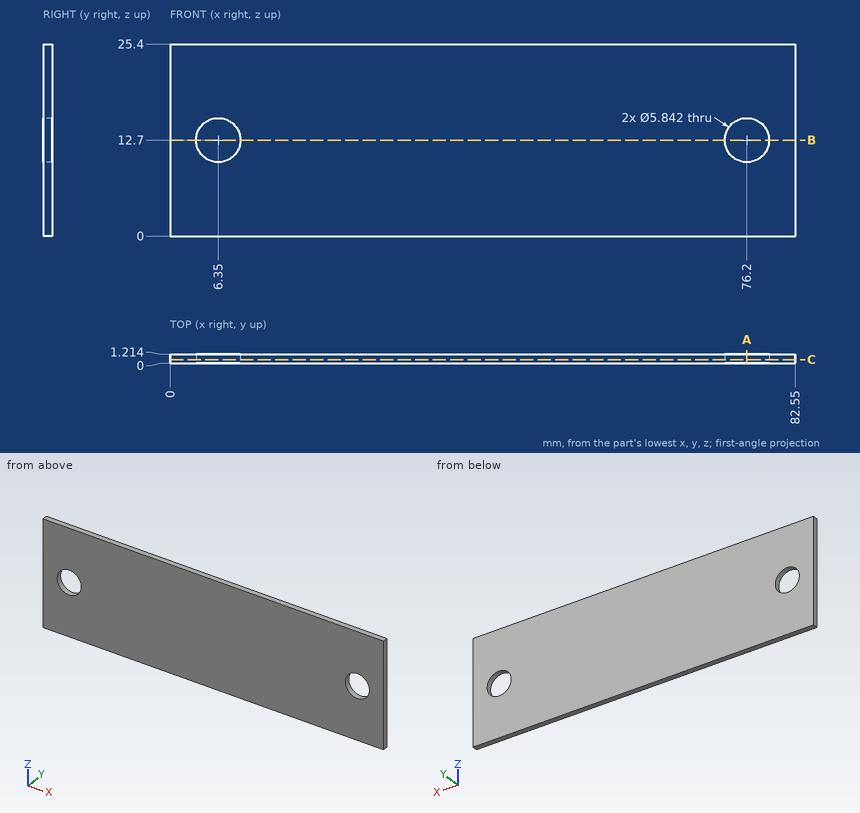
The drawing under review shows one solid part. Ordinate dimensions are in mm from its lowest x, y, z. Round coordinates to 2 decimals unless told otherwise and drop trailing zeros. Order: outer loops, then holes, each group sorted by start corner. A loop starts at its lowest first (then second) coordinate and runs counter-clockwise, first axis right, second up. Notation, with made-up numbers: M 61.25,7 L 110.25,7 A21 ccw 110.25,40 Z; hole C -35.75,-38.75 d6. An arc over 180 degrees is marked long. Answer as CSV lines item,"result". Start each with the question number.
1) Add section C-C (y = 0.5). Give the boundary of the cut face in (x, z), then the cut area to 3 significant figures.
2) Add section B-B (z = 12.7). Give the boundary of the cut face in (x, y).
3) For pin 1 Ø3.5 at (x, z) = (6.35, 12.7) entering from +Y, flat-tipped, find the tip position at first contact; note if it passes through.
4) Wall thickness on line 1 along X through (y, z) = (0.6, 12.7); line 2 along X through (y, z) = (1, 13.5): over which ranges is each line inside the solid? List them lowest first. Write a range as [from, to].
5) Add section A-A (x = 76.2). Give the boundary of the cut face in (y, z).
Resolved:
1,outline,"M 0,0 L 82.55,0 L 82.55,25.4 L 0,25.4 Z; hole C 6.35,12.7 d5.84; hole C 76.2,12.7 d5.84"
1,area,"2,040 mm^2"
2,outline,"M 0,0 L 3.43,0 L 3.43,1.21 L 0,1.21 Z; M 9.27,0 L 73.28,0 L 73.28,1.21 L 9.27,1.21 Z; M 79.12,0 L 82.55,0 L 82.55,1.21 L 79.12,1.21 Z"
3,pin 1,"through"
4,line 1,"[0, 3.43], [9.27, 73.28], [79.12, 82.55]"
4,line 2,"[0, 3.54], [9.16, 73.39], [79.01, 82.55]"
5,outline,"M 0,0 L 1.21,0 L 1.21,9.78 L 0,9.78 Z; M 0,15.62 L 1.21,15.62 L 1.21,25.4 L 0,25.4 Z"
